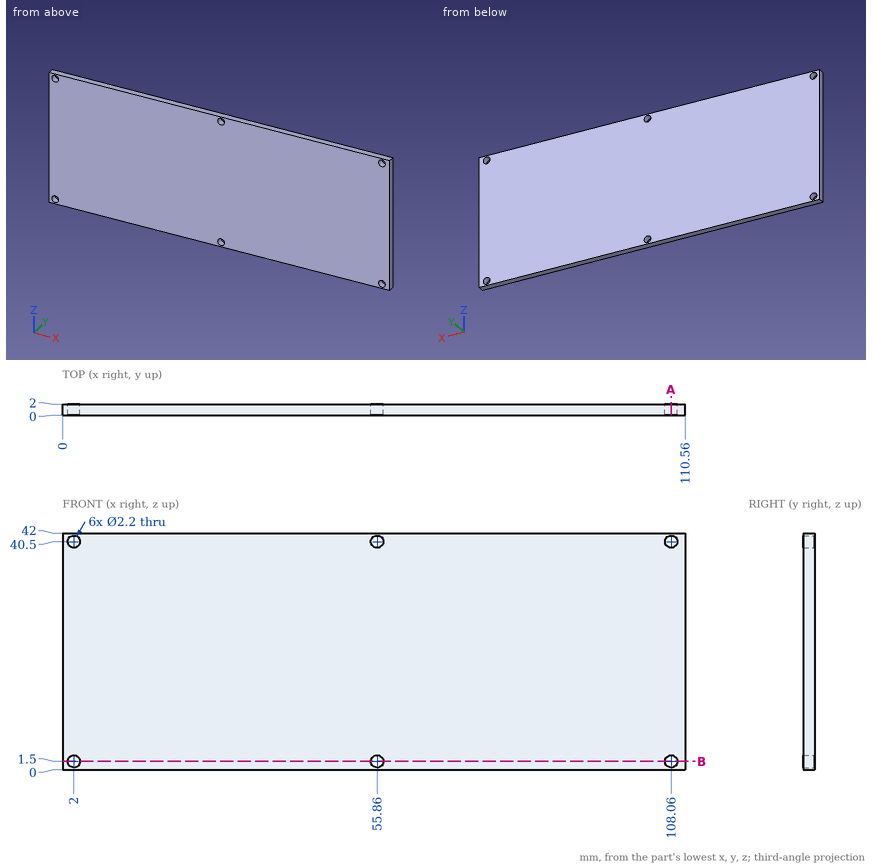
Can you work these out from the drawing? Everything is in mm from the part's minimum corner. Give positions to 0.01 mm unless a question says otherwise; leave off trailing zeros. Order: outer loops, then holes, each group sorted by start corner. A loop starts at its lowest first (then second) coordinate and runs counter-clockwise, first axis right, second up. Notation, with made-up numbers: M 48.5,53.5 L 86.5,53.5 A22 cw 86.5,75.5 Z; hole C -38,-30.5 d7. An arc over 180 degrees is marked long. One line per item, written item: value.
Item 1: For pin 1 (2 mm diameter, centred on x = 2, z = 1.5, fed in from +Y); pin 2 (3.5 mm diameter, centred on x = 55.86, z = 1.5, fed in from +Y), each with a flat end and sliding along its axis, tell me the tip position at first contact or that it passes through.
Verdict:
pin 1: through
pin 2: y = 2
Item 2: If we section it at B-B on z = 1.5: Write out the boundary of the cut face in (x, y).
Verdict:
outline: M 0,0 L 0.9,0 L 0.9,2 L 0,2 Z; M 3.1,0 L 54.76,0 L 54.76,2 L 3.1,2 Z; M 56.96,0 L 106.96,0 L 106.96,2 L 56.96,2 Z; M 109.16,0 L 110.56,0 L 110.56,2 L 109.16,2 Z
Item 3: Please list where these lines run through material, in increasing order: line 1 (X direction, y = 1.3, z = 40.5); line 2 (Z direction, x = 2, y = 1.65).
Verdict:
line 1: 0 to 0.9, 3.1 to 54.76, 56.96 to 106.96, 109.16 to 110.56
line 2: 0 to 0.4, 2.6 to 39.4, 41.6 to 42
Item 4: If we section it at A-A on x = 108.06: Write out the boundary of the cut face in (y, z).
Verdict:
outline: M 0,0 L 2,0 L 2,0.4 L 0,0.4 Z; M 0,2.6 L 2,2.6 L 2,39.4 L 0,39.4 Z; M 0,41.6 L 2,41.6 L 2,42 L 0,42 Z
